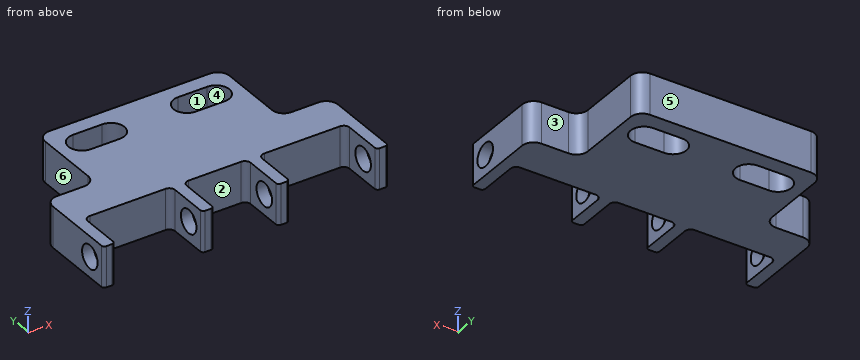
Autodesk Inventor part; units mm, degrees
ref_plane "YZ Plane" through (0, 0, 0) normal (1, 0, 0) x (0, 1, 0)
ref_plane "XZ Plane" through (0, 0, 0) normal (0, 1, 0) x (-1, 0, 0)
ref_plane "XY Plane" through (0, 0, 0) normal (0, 0, 1) x (1, 0, 0)
sketch "Sketch1" plane through (0, 0, 0) normal (0, 0, 1) x (1, 0, 0)
  line L0 (0, 0) -> (49, 0)
  line L1 (49, 0) -> (49, 30)
  line L2 (49, 30) -> (0, 30)
  line L3 (0, 30) -> (0, 0)
  dimension "d0" = 30
  dimension "d1" = 49
extrude "Extrusion1" add sketch "Sketch1" along normal blind 7
sketch "Sketch2" plane through (0, 0, 7) normal (0, 0, 1) x (1, 0, 0)
  arc A0 (12.975, 27.3) -> (12.975, 22.7) centre (12.975, 25) ccw
  arc A1 (17.975, 22.7) -> (17.975, 27.3) centre (17.975, 25) ccw
  arc A2 (31.025, 27.3) -> (31.025, 22.7) centre (31.025, 25) ccw
  arc A3 (36.025, 22.7) -> (36.025, 27.3) centre (36.025, 25) ccw
  line L0 (12.975, 27.3) -> (17.975, 27.3)
  line L1 (12.975, 22.7) -> (17.975, 22.7)
  line L2 (31.025, 27.3) -> (36.025, 27.3)
  line L3 (31.025, 22.7) -> (36.025, 22.7)
  line L4 (49, 30) -> (0, 30)
  line L5 (0, 30) -> (0, 0)
  dimension "d4" = 4.6
  dimension "d5" = 4.6
  dimension "d6" = 4.6
  dimension "d8" = 5
  dimension "d9" = 5
  dimension "d10" = 13.05
  dimension "d11" = 5
  dimension "d12" = 12.975
  dimension "d13" = 49
  dimension "d17" = 2.3
extrude "Extrusion2" cut sketch "Sketch2" against normal up to next
sketch "Sketch3" plane through (0, 0, 7) normal (0, 0, 1) x (1, 0, 0)
  arc A0 (12.975, 27.3) -> (12.975, 22.7) centre (12.975, 25) ccw
  line L0 (12.975, 27.3) -> (17.975, 27.3)
  arc A1 (17.975, 22.7) -> (17.975, 27.3) centre (17.975, 25) ccw
  line L1 (17.975, 22.7) -> (12.975, 22.7)
  arc A2 (31.025, 27.3) -> (31.025, 22.7) centre (31.025, 25) ccw
  line L2 (31.025, 27.3) -> (36.025, 27.3)
  arc A3 (36.025, 22.7) -> (36.025, 27.3) centre (36.025, 25) ccw
  line L3 (36.025, 22.7) -> (31.025, 22.7)
  line L4 (0, 0) -> (49, 0)
  line L5 (49, 0) -> (49, 30)
  line L6 (49, 30) -> (0, 30)
  line L7 (0, 30) -> (0, 0)
  line L8 (2, 8) -> (17, 8)
  line L9 (17, 8) -> (17, 0)
  line L10 (17, 0) -> (2, 0)
  line L11 (2, 0) -> (2, 8)
  line L12 (32, 8) -> (47, 8)
  line L13 (47, 8) -> (47, 0)
  line L14 (47, 0) -> (32, 0)
  line L15 (32, 0) -> (32, 8)
  line L16 (0, 0) -> (49, 0)
  line L17 (19, 0) -> (30, 0)
  line L18 (30, 0) -> (30, 8)
  line L19 (30, 8) -> (19, 8)
  line L20 (19, 8) -> (19, 0)
  dimension "d18" = 8
  dimension "d19" = 15
  dimension "d20" = 15
  dimension "d21" = 15
  dimension "d22" = 2
  dimension "d23" = 49
  dimension "d35" = 2
  dimension "d36" = 2
sketch "Sketch4" plane through (0, 0, 7) normal (0, 0, 1) x (1, 0, 0)
  arc A0 (12.975, 27.3) -> (12.975, 22.7) centre (12.975, 25) ccw
  line L0 (12.975, 27.3) -> (17.975, 27.3)
  arc A1 (17.975, 22.7) -> (17.975, 27.3) centre (17.975, 25) ccw
  line L1 (17.975, 22.7) -> (12.975, 22.7)
  arc A2 (31.025, 27.3) -> (31.025, 22.7) centre (31.025, 25) ccw
  line L2 (31.025, 27.3) -> (36.025, 27.3)
  arc A3 (36.025, 22.7) -> (36.025, 27.3) centre (36.025, 25) ccw
  line L3 (36.025, 22.7) -> (31.025, 22.7)
  line L4 (0, 0) -> (49, 0)
  line L5 (49, 0) -> (49, 30)
  line L6 (49, 30) -> (0, 30)
  line L7 (0, 30) -> (0, 0)
  line L8 (0, 30) -> (8.675, 30)
  line L9 (8.675, 30) -> (8.675, 15)
  line L10 (8.675, 15) -> (0, 15)
  line L11 (0, 15) -> (0, 30)
  line L12 (49, 30) -> (40.325, 30)
  line L13 (40.325, 30) -> (40.325, 15)
  line L14 (40.325, 15) -> (49, 15)
  line L15 (49, 15) -> (49, 30)
  dimension "d26" = 8.675
  dimension "d27" = 8.675
  dimension "d28" = 30
  dimension "d29" = 15
  dimension "d31" = 2.3
  dimension "d32" = 12.975
extrude "Extrusion3" cut sketch "Sketch3" against normal up to next contours L11 L8 L9 L4 | L20 L19 L18 L4 | L4 L15 L12 L13
extrude "Extrusion4" cut sketch "Sketch4" against normal up to next contours L7 L6 L9 L10 | L14 L13 L6 L5
sketch "Sketch5" plane through (49, 0, 7) normal (1, 0, 0) x (0, 0, -1)
  circle A0 centre (3.5, 3.5) radius 2
  line L0 (0, 0) -> (0, 15)
  line L1 (7, 0) -> (0, 0)
  dimension "d37" = 4
  dimension "d38" = 3.5
  dimension "d39" = 3.5
  dimension "d40" = 7
extrude "Extrusion5" cut sketch "Sketch5" against normal through all
fillet "Fillet1" radius 1 6 edges at (2, 8, 3.5) (17, 8, 3.5) (19, 8, 3.5) (30, 8, 3.5) (32, 8, 3.5) (47, 8, 3.5)
fillet "Fillet2" radius 2 6 edges at (40.325, 15, 3.5) (8.675, 15, 3.5) (8.675, 30, 3.5) (40.325, 30, 3.5) (49, 15, 3.5) (0, 15, 3.5)
fillet "Fillet3" radius 0.5 8 edges at (0, 0, 3.5) (2, 0, 3.5) (17, 0, 3.5) (19, 0, 3.5) (30, 0, 3.5) (32, 0, 3.5) (47, 0, 3.5) (49, 0, 3.5)
equation "\"d5\" = d4"
equation "\"d6\" = d4"
equation "\"d12\" = -0.5 * d8 - 0.5 * d9 + 0.5 * d13 - 0.5 * d10"
equation "\"d17\" = 0.5 * d6"
equation "\"d22\" = -0.5 * d20 - 0.5 * d19 + 0.5 * d23 - 0.5 * d21"
equation "\"d35\" = d22"
equation "\"d36\" = d35"
equation "\"d26\" = d27"
equation "\"d38\" = 0.5 * d40"
equation "\"d39\" = d38"
properties part number "tubing_connection_holder"
Design review of the part built by this model. Coordinates are the model's own, in mm. Face numbers are marked on the shaded views. A direction names the side the tool comes from. Round coordinates to 2 decimals unless told otherwise and drop trailing zeros. Write each loop counter-clockwise with the first axis right and the second up, starting at its lowest first coordinate (ties: lowest second). Pieces come first, ordered by that corner, then holes. Notation, with made-up numbers: M -9.5,-24 L 22.5,-24 A20 ccw 22.5,-17 Z; hole C -29.5,4.25 d2. An arc over 180 degrees is marked long. One line per item, written item: value. Start each with the question number.
1. To check wall thickness, follow probe 1 along X at (y, z) = (1.5, 2); probe 2 along Y at (x, z) = (17.65, 3.5); probe 3 along Y at (x, z) = (13, 3.25). State the ranges of each line that lie inside material, in increasing order. Write a range as from..to.
2. Take a section at A-A on y = 3.5. State how many separate pieces and enclosed holes the cut face has, then the cut area to 3 significant figures.
3. Take a section at B-B on y = 25. State the section outline as (x, z) points (3 decimals).
4. Clearance check with flat-ended pins moving along their axes: P1, Ø2, axis at x = 38.5, z = 3.5, coming from the -Y side; P2, Ø1, axis at y = 20.5, z = 5, coming from the -X side (3 decimals); P3, Ø2.5, axis at x = 16, z = 4.5, coming from the -Y side. State where each tip first meets the part, or that it passes through.
5. Draft analysis for pull direction X (two halves, no side actions). For the marked faces 4, 5 and 6, state which applies: pulls with the +X half, pulls with the -X half, needs draft (parallel to the pull), parting line crosses it, or undercut.
6. For the marked faces 1, 2 and 3, list the 3-axis set-ups (+Z, -Z, +X, -X, +Y, -Y) from which the entire face can be reached by the end or side of a thin tool; tool diameter is ignored.
Computed:
1. probe 1: x = 0..2, 17..19, 30..32, 47..49
1. probe 2: y = 0..1.5, 5.5..22.7, 27.3..30
1. probe 3: y = 8..22.7, 27.3..30
2. separate pieces: 8
2. enclosed holes: 0
2. area: 24.0 mm²
3. outline: M 8.675,0 L 10.675,0 L 10.675,7 L 8.675,7 Z; M 20.275,0 L 28.725,0 L 28.725,7 L 20.275,7 Z; M 38.325,0 L 40.325,0 L 40.325,7 L 38.325,7 Z
4. P1: stops at y = 8
4. P2: stops at x = 8.675
4. P3: stops at y = 0.07
5. face 4: undercut
5. face 5: needs draft
5. face 6: pulls with the -X half
6. face 1: +Z, -Z
6. face 2: +Z, -Z, -Y
6. face 3: +Z, -Z, +X, +Y
